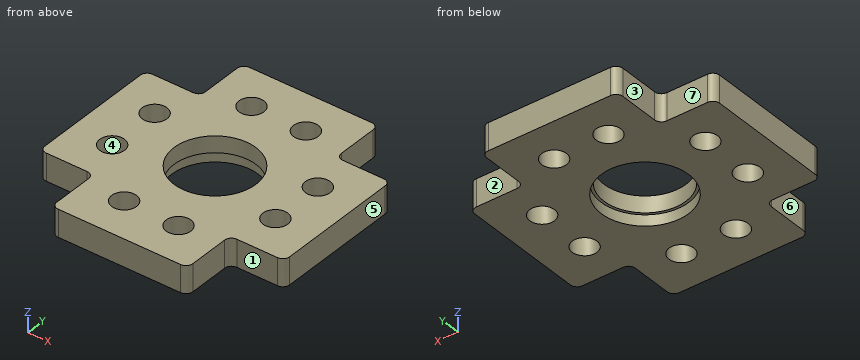
```python
from build123d import *

# Parameters (mm, degrees)
SKETCH_1_R               = 15.04
EXTRUDE_1_DEPTH          = 10
FILLET_1_R               = 2.5
SKETCH_2_R               = 16.04
CUT_EXTRUDE_1_DEPTH      = 4
FILLET_2_R               = 2.5
SKETCH_5_R               = 4.55
CUT_EXTRUDE_2_DEPTH      = 76.6565237
PATTERN_CIRCULAR_1_COUNT = 4


with BuildPart() as part:
    # 스케치1 → 보스-돌출1 (new body)
    with BuildSketch(Plane.XY):
        Polygon((-30.009087535, 25), (-10.009087535, 25), (-10.009087535, 45), (39.990912465, 45), (39.990912465, 25), (59.990912465, 25), (59.990912465, -25), (39.990912465, -25), (39.990912465, -45), (-10.009087535, -45), (-10.009087535, -25), (-30.009087535, -25), align=None)
        with Locations((14.990912465, 0)):
            Circle(SKETCH_1_R, mode=Mode.SUBTRACT)
    extrude(amount=EXTRUDE_1_DEPTH)

    # 필렛1
    fillet_1_edges = [part.edges().sort_by_distance(p)[0] for p in [
        (-10.009087535, 25, 5),
        (39.990912465, 25, 5),
        (39.990912465, -25, 5),
        (-10.009087535, -25, 5),
    ]]
    fillet(fillet_1_edges, radius=FILLET_1_R)

    # 스케치2 → 컷-돌출1 (cut)
    with BuildSketch(Plane(origin=(0, 0, 0), x_dir=(-1, 0, 0), z_dir=(0, 0, -1))):
        with Locations((-14.990912465, 0)):
            Circle(SKETCH_2_R)
    extrude(amount=-CUT_EXTRUDE_1_DEPTH, mode=Mode.SUBTRACT)

    # 필렛2
    fillet_2_edges = [part.edges().sort_by_distance(p)[0] for p in [
        (-30.009087535, 25, 5),
        (-10.009087535, 45, 5),
        (39.990912465, 45, 5),
        (59.990912465, 25, 5),
        (59.990912465, -25, 5),
        (39.990912465, -45, 5),
        (-10.009087535, -45, 5),
        (-30.009087535, -25, 5),
    ]]
    fillet(fillet_2_edges, radius=FILLET_2_R)

    # 스케치5 → 컷-돌출2 (cut, through all)
    with BuildSketch(Plane.XY.offset(10)):
        with Locations((-15.009087535, -10)):
            Circle(SKETCH_5_R)
        with Locations((-15.009087535, 10)):
            Circle(SKETCH_5_R)
    cut_extrude_2 = extrude(amount=-CUT_EXTRUDE_2_DEPTH, mode=Mode.SUBTRACT)

    # 원형 패턴1: 컷-돌출2 ×4 about axis
    pattern_circular_1_axis = Axis((14.990912465, 0, 0), (0, 0, 1))
    for i in range(1, PATTERN_CIRCULAR_1_COUNT):
        add(cut_extrude_2.rotate(pattern_circular_1_axis, i * 360 / PATTERN_CIRCULAR_1_COUNT), mode=Mode.SUBTRACT)


solid = part.part
```
Check sheet for the modelled part. Datum: model origin and axes. Units: mm. Face numbers are marked on the shaded views. A direction names the side the tool comes from. Round coordinates to 2 decimals unless told otherwise and drop trailing zeros. Order: outer loops, then holes, each group sorted by start corner. A loop starts at its lowest first (then second) coordinate and runs counter-clockwise, first axis right, second up. Notation, with made-up numbers: (37, 55.5) -> (54, 55.5) arc R17 ccw to (54, 76.5) -> close; hole circle Ø8 at (16, 21.5). An arc over 180 degrees is marked (long way). Use CSV: the item, a comma, the result in double quotes.
(1) Tool access check on the marked faces 1, 2 and 3. Record the directions out of +Z, -Z, +X, -X, +Y, -Y that give a thin tool (end or side, any length) a straight path to the whole face; none if there is none.
Worked out:
face 1,"+Z, -Z, +X, -Y"
face 2,"+Z, -Z, +X, +Y"
face 3,"+Z, -Z, -X, +Y"
(2) Cross-section at A-A (y = -30). Record the boundary of the cut face in (x, z), and give its area (3 significant figures).
Worked out:
outline,"(-10.01, 0) -> (0.44, 0) -> (0.44, 10) -> (-10.01, 10) -> close; (9.54, 0) -> (20.44, 0) -> (20.44, 10) -> (9.54, 10) -> close; (29.54, 0) -> (39.99, 0) -> (39.99, 10) -> (29.54, 10) -> close"
area,"318 mm²"
(3) Draft check along X on the marked faces 4, 5, 6 and 7. Enter one of: pulls with the +X half, pulls with the -X half, needs draft (parallel to the pull), parting line crosses it, or undercut.
Worked out:
face 4,"undercut"
face 5,"pulls with the +X half"
face 6,"pulls with the -X half"
face 7,"needs draft"
(4) Cross-section at C-C (y = 0). Record the boundary of the cut face in (x, z), and give its area (3 significant figures).
Worked out:
outline,"(-30.01, 0) -> (-1.05, 0) -> (-1.05, 4) -> (-0.05, 4) -> (-0.05, 10) -> (-30.01, 10) -> close; (30.03, 4) -> (31.03, 4) -> (31.03, 0) -> (59.99, 0) -> (59.99, 10) -> (30.03, 10) -> close"
area,"591 mm²"
(5) Depth check by flat-ended pin: pin 1 (4 mm diameter, centred on y = -34.5, z = 4, fed in from -X); pin 2 (5 mm diameter, centred on x = -16.5, z = 5.5, fed in from +Y); pin 3 (3 mm diameter, centred on y = -34.5, z = 2.5, fed in from +X). Enter the tip coordinate at first touch or a pass-through.
Worked out:
pin 1,"x = -10.01"
pin 2,"y = 25"
pin 3,"x = 39.99"
(6) Cross-section at D-D (z = 2.75). Count the separate pieces of the cut face and the enclosed holes in it, and give its area (3 significant figures).
Worked out:
separate pieces,"1"
enclosed holes,"9"
area,"5,170 mm²"
(7) Cross-section at B-B (x = 46). Record the boundary of the cut face in (y, z), and give its area (3 significant figures).
Worked out:
outline,"(-25, 0) -> (-14.44, 0) -> (-14.44, 10) -> (-25, 10) -> close; (-5.56, 0) -> (5.56, 0) -> (5.56, 10) -> (-5.56, 10) -> close; (14.44, 0) -> (25, 0) -> (25, 10) -> (14.44, 10) -> close"
area,"323 mm²"
(8) Material ranges on line 1 along Y through (x, z) = (28, 8.75); line 2 along X through (y, z) = (-30, 7.5); line 3 along X through (y, z) = (30.5, 1.75), recorded low to high. Write a range as from..to.
Worked out:
line 1,"-45..-33.41, -26.59..-7.55, 7.55..26.59, 33.41..45"
line 2,"-10.01..0.44, 9.54..20.44, 29.54..39.99"
line 3,"-10.01..0.47, 9.51..20.47, 29.51..39.99"
